Part print with two shaded views. Sizes in mm from the minimum x, y, z corner. A direction names the side the tool comes from. Coordinates: 2 decimals unless noted, no trailing zeros. Write each loop counter-clockwise with the first axis right and the second up, starting at its lowest first coordinate (ties: lowest second). Pieces come first, ordered by that corner, then holes. Notation, with made-up numbers: (-37, -23.75) - (-13, -23.75) arc R11 ccw to (-13, -9.75) - close; hole circle Ø9 at (30, 22). An arc over 180 degrees is marked (long way). Answer in a Markdown table with one row per item. Add a question column.
Q1. Two-plate mould, pull along X, no slides. Class the marked faces 1, 2, 3 and 4: +X half, -X half, draft (parallel to the pull), parting line (faces both ways), or undercut.
Q2. Band-saw the part on C-C (y = 18.5). List the corners of the cut face in (x, z).
Q3. Drill centre lines: line 1 along Y through (x, z) = (3, 1.4); line 2 along X through (y, z) = (4.25, 1.55); line 3 along Y through (x, z) = (5, 0.45). Where is each one in solid material? Low to high. Write a range as from..to.
Q4. Band-saw the part on A-A (x = 3). List the corners of the cut face in (y, z), and give its area (3 significant figures).
Q5. Band-saw the part on D-D (y = 3.5). List the corners of the cut face in (x, z).
Q6. 3-axis set-ups, long thin cutter, end or side, ignore diameter. For the marked faces 5, 6 and 7: which of +Z, -Z, +X, -X, +Y, -Y reach the whole face in a straight line?
Q7. Band-saw the part on B-B (z = 0.9). List the corners of the cut face in (x, y).
Q8. Pin check, flat tips, straight feed: pin 1 (3 mm diameter, centred on x = 3, y = 19, fed in from +Z); pin 2 (1.6 mm diameter, centred on x = 37, z = 1.5, fed in from -Y); pin 3 (1.6 mm diameter, centred on x = 3, y = 12, fed in from +Z). Stop position of each tip, or through.
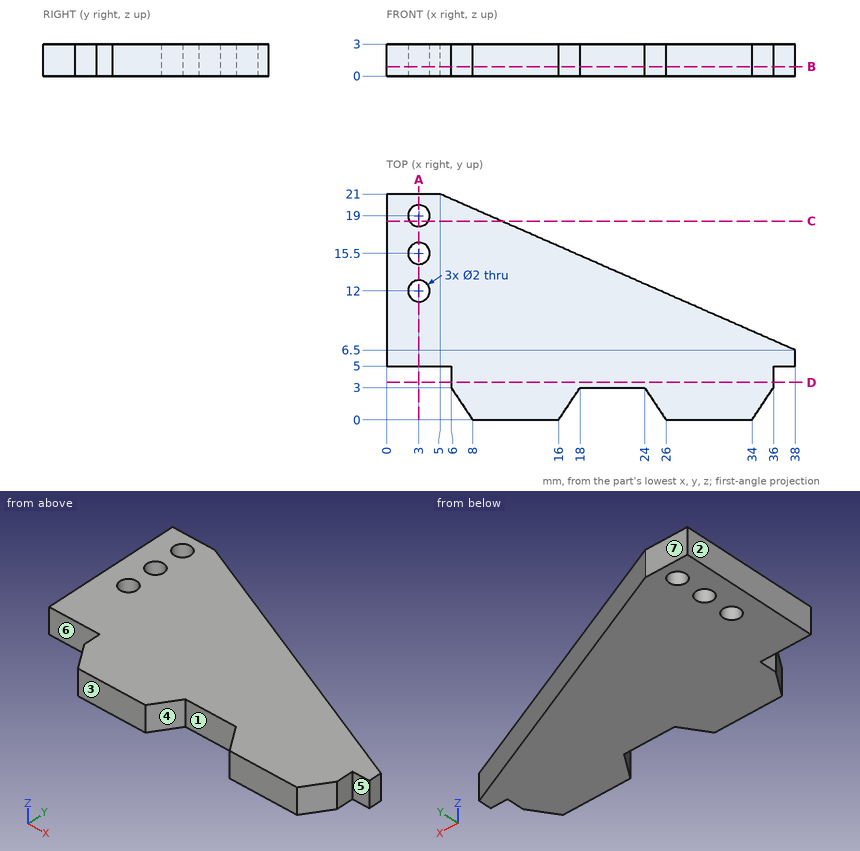
Checked values:
| question | item | result |
|---|---|---|
| 1 | face 1 | undercut |
| 1 | face 2 | -X half |
| 1 | face 3 | draft |
| 1 | face 4 | undercut |
| 2 | outline | (0, 0) - (2.13, 0) - (2.13, 3) - (0, 3) - close; (3.87, 0) - (10.69, 0) - (10.69, 3) - (3.87, 3) - close |
| 3 | line 1 | y = 5..11, 13..14.5, 16.5..18, 20..21 |
| 3 | line 2 | x = 6..36 |
| 3 | line 3 | y = 5..21 |
| 4 | outline | (5, 0) - (11, 0) - (11, 3) - (5, 3) - close; (13, 0) - (14.5, 0) - (14.5, 3) - (13, 3) - close; (16.5, 0) - (18, 0) - (18, 3) - (16.5, 3) - close; (20, 0) - (21, 0) - (21, 3) - (20, 3) - close |
| 4 | area | 30.0 mm² |
| 5 | outline | (6, 0) - (36, 0) - (36, 3) - (6, 3) - close |
| 6 | face 5 | +Z, -Z, +X, -Y |
| 6 | face 6 | +Z, -Z, -X, -Y |
| 6 | face 7 | +Z, -Z, +X, -X, +Y |
| 7 | outline | (0, 5) - (6, 5) - (6, 3) - (8, 0) - (16, 0) - (18, 3) - (24, 3) - (26, 0) - (34, 0) - (36, 3) - (36, 5) - (38, 5) - (38, 6.5) - (5, 21) - (0, 21) - close; hole circle Ø2 at (3, 12); hole circle Ø2 at (3, 15.5); hole circle Ø2 at (3, 19) |
| 8 | pin 1 | stops at z = 3 |
| 8 | pin 2 | stops at y = 5 |
| 8 | pin 3 | passes through |
